Autodesk Fusion 360 part; units mm, degrees
sketch "Sketch1" plane through (0, 0, 0) normal (0, 0, 1) x (1, 0, 0) in component "Upper Layer"
  line L0 (30, -35) -> (-30, -35)
  line L1 (-30, -35) -> (-30, 35)
  line L2 (-30, 35) -> (30, 35)
  line L3 (30, 35) -> (30, -35)
  line L4 (30, -35) -> (-30, 35) construction
  line L5 (-30, -35) -> (30, 35) construction
  line L6 (28, -38) -> (-28, -38)
  line L7 (-33, -33) -> (-33, 33)
  line L8 (-28, 38) -> (28, 38)
  line L9 (33, 33) -> (33, -33)
  line L10 (33, -38) -> (-33, 38) construction
  line L11 (-33, -38) -> (33, 38) construction
  arc A0 (-28, 38) -> (-33, 33) centre (-28, 33) ccw
  arc A1 (33, 33) -> (28, 38) centre (28, 33) ccw
  arc A2 (-33, -33) -> (-28, -38) centre (-28, -33) ccw
  arc A3 (28, -38) -> (33, -33) centre (28, -33) ccw
  dimension "d1" = 60
  dimension "d2" = 70
  dimension "d3" = 66
  dimension "d4" = 76
  dimension "d51" = 5
  dimension "d52" = 5
  dimension "d53" = 5
  dimension "d54" = 5
extrude "Extrude1" add sketch "Sketch1" along normal blind 3 contours L0 L1 L2 L3 | L6 L7 L8 L9 A0 A1 A2 A3 in component "Upper Layer"
sketch "Sketch2" plane through (0, 0, 3) normal (0, 0, 1) x (-1, 0, 0) in component "Upper Layer"
  line L0 (-28, -38) -> (28, -38)
  line L1 (33, -33) -> (33, 33)
  line L2 (28, 38) -> (-28, 38)
  line L3 (-33, 33) -> (-33, -33)
  line L4 (-30, 35) -> (30, 35)
  line L5 (30, 35) -> (30, -35)
  line L6 (30, -35) -> (-30, -35)
  line L7 (-30, -35) -> (-30, 35)
  line L8 (-30, 35) -> (30, -35) construction
  line L9 (30, 35) -> (-30, -35) construction
  line L10 (0, 35) -> (0, -35) construction
  line L11 (2.5, -11) -> (-2.5, -11)
  line L12 (-2.5, -11) -> (-2.5, -20)
  line L13 (-2.5, -20) -> (2.5, -20)
  line L14 (2.5, -20) -> (2.5, -11)
  line L15 (2.5, -11) -> (-2.5, -20) construction
  line L16 (-2.5, -11) -> (2.5, -20) construction
  line L17 (0, -11) -> (0, 9) construction
  line L18 (0, 9) -> (-7.5, 9) construction
  line L19 (-7.5, 9) -> (-15.5, 9)
  line L20 (-15.5, 9) -> (-15.5, 4)
  line L21 (-15.5, 4) -> (-7.5, 4)
  line L22 (-7.5, 4) -> (-7.5, 9)
  line L23 (15.5, 4) -> (7.5, 4)
  line L24 (7.5, 4) -> (7.5, 9)
  line L25 (15.5, 9) -> (15.5, 4)
  line L26 (7.5, 9) -> (15.5, 9)
  line L27 (-5.5, -8) -> (5.5, -8)
  line L28 (5.5, -8) -> (5.5, -23)
  line L29 (5.5, -23) -> (-5.5, -23)
  line L30 (-5.5, -23) -> (-5.5, -8)
  line L31 (-5.5, -8) -> (5.5, -23) construction
  line L32 (5.5, -8) -> (-5.5, -23) construction
  line L33 (-11.5, 9) -> (-11.5, 4) construction
  line L34 (-7.5, 6.5) -> (-15.5, 6.5) construction
  line L35 (-19, 11.5) -> (-4, 11.5)
  line L36 (-4, 11.5) -> (-4, 1.5)
  line L37 (-4, 1.5) -> (-19, 1.5)
  line L38 (-19, 1.5) -> (-19, 11.5)
  line L39 (-19, 11.5) -> (-4, 1.5) construction
  line L40 (-4, 11.5) -> (-19, 1.5) construction
  line L41 (4, 1.5) -> (19, 1.5)
  line L42 (4, 11.5) -> (4, 1.5)
  line L43 (19, 11.5) -> (4, 11.5)
  line L44 (19, 1.5) -> (19, 11.5)
  arc A0 (33, 33) -> (28, 38) centre (28, 33) ccw
  arc A1 (-28, 38) -> (-33, 33) centre (-28, 33) ccw
  arc A2 (-33, -33) -> (-28, -38) centre (-28, -33) ccw
  arc A3 (28, -38) -> (33, -33) centre (28, -33) ccw
  point P0 (0, -15.5)
  point P1 (0, -15.5)
  point P2 (-11.5, 6.5)
  dimension "d7" = 5
  dimension "d8" = 9
  dimension "d9" = 20
  dimension "d10" = 7.5
  dimension "d11" = 8
  dimension "d12" = 5
  dimension "d13" = 11
  dimension "d14" = 15
  dimension "d15" = 15
  dimension "d16" = 10
extrude "Extrude2" cut sketch "Sketch2" against normal up to surface (3 mm away) contours L11 L12 L13 L14 in component "Upper Layer"
extrude "Extrude3" add sketch "Sketch2" along normal blind 3 contours L27 L28 L29 L30 in component "Upper Layer"
extrude "Extrude4" cut sketch "Sketch2" against normal up to surface (3 mm away) contours L19 L20 L21 L22 | L23 L24 L25 L26 in component "Upper Layer"
extrude "Extrude5" add sketch "Sketch2" along normal blind 3 contours L35 L36 L37 L38 | L41 L42 L43 L44 in component "Upper Layer"
sketch "Sketch2 (2)" plane through (0, 0, -8.9199) normal (0, 0, -1) x (1, 0, 0)
  line L0 (22.45, -32.5) -> (22.45, -27.6)
  line L1 (22.45, -27.6) -> (17.55, -27.6)
  line L2 (17.55, -27.6) -> (17.55, -32.5)
  line L3 (17.55, -32.5) -> (22.45, -32.5)
  line L4 (-17.55, -32.45) -> (-17.55, -27.55)
  line L5 (-17.55, -27.55) -> (-22.45, -27.55)
  line L6 (-22.45, -27.55) -> (-22.45, -32.45)
  line L7 (-22.45, -32.45) -> (-17.55, -32.45)
sketch "Sketch4" plane through (0, 0, 3) normal (0, 0, 1) x (1, 0, 0) in component "Upper Layer"
  line L0 (0, 30) -> (-18, 30) construction
  circle A0 centre (-18, 30) radius 3
  line L1 (-18, 30) -> (-15, 30)
  line L2 (-18, 30) -> (-7.5877, 30) construction
  line L3 (-18, 30) -> (18, 30) construction
  circle A1 centre (18, 30) radius 3
  dimension "d37" = 6
  dimension "d38" = 36
  dimension "d39" = 6
  dimension "d50" = 18
extrude "Extrude9" cut sketch "Sketch4" against normal up to surface (3 mm away) in component "Upper Layer"
sketch "Sketch3" plane through (0, 0, 3) normal (0, 0, 1) x (-1, 0, 0)
  line L0 (30, 35) -> (27.5, 35) construction
  line L1 (30, 35) -> (30, 32.5) construction
  circle A0 centre (27.5, 32.5) radius 2.5
  line L2 (40, 0) -> (-40, 0)
  line L3 (0, -45) -> (0, 47.452)
  circle A1 centre (27.5, -32.5) radius 2.5
  circle A2 centre (-27.5, -32.5) radius 2.5
  circle A3 centre (-27.5, 32.5) radius 2.5
  circle A4 centre (27.5, -32.5) radius 1.5
  circle A5 centre (27.5, 32.5) radius 1.5
  circle A6 centre (-27.5, -32.5) radius 1.5
  circle A7 centre (-27.5, 32.5) radius 1.5
  dimension "d42" = 2.5
  dimension "d43" = 2.5
  dimension "d44" = 3
  dimension "d45" = 3
  dimension "d46" = 3
  dimension "d47" = 3
extrude "Extrude10" cut sketch "Sketch3" against normal blind 3 contours A4 | A5 | A6 | A7 in component "Upper Layer"
component "Upper Layer" placed x (1, 0, 0) y (0, 1, 0) z (0, 0, 1) at (0, 0, 0)
equation "d10 = ( 15 / 2 ) * 1 mm"
Part model, mm, in its own coordinate system. A direction names the side the tool comes from. Round coordinates to 2 decimals unless told otherwise and drop trailing zeros. Write each loop counter-clockwise with the first axis right and the second up, starting at its lowest first coordinate (ties: lowest second). Pieces come first, ordered by that corner, then holes.
Item 1: Probe L1, parallel to X at y = -5.5, z = 5.5; L2, parallel to Y at x = -27.5, z = 0.9; L3, parallel to X at y = 19, z = 3.7. List the from-to ranges inside material, lowest first.
Results:
L1: x = -19 to -15.5, -7.5 to -4, 4 to 7.5, 15.5 to 19
L2: y = -38 to -34, -31 to 31, 34 to 38
L3: x = -5.5 to -2.5, 2.5 to 5.5
Item 2: Cut at C-C, the plane y = 30. Give the cut face in (x, z), plus the area to 3 significant figures.
Results:
outline: (-33, 0) - (-21, 0) - (-21, 3) - (-33, 3) - close; (-15, 0) - (15, 0) - (15, 3) - (-15, 3) - close; (21, 0) - (33, 0) - (33, 3) - (21, 3) - close
area: 162 mm2
Item 3: Two-plate mould, pull along X, no slides. Class faces 1 (the flat face through (0, 38, 1)), 2 (the cylindrical face through (-26.3, 33.4, 1.5)), 3 (the cylindrical face through (-26.3, -31.6, 1.5)), 4 (the flat face through (5.5, 16, 4)): +X half, -X half, draft (parallel to the pull), parting line (faces both ways), or undercut.
Results:
face 1: draft
face 2: undercut
face 3: undercut
face 4: +X half
Item 4: Cut at A-A, the plane x = 18. Give the cut face in (y, z), plus the area to 3 significant figures.
Results:
outline: (-38, 0) - (27, 0) - (27, 3) - (-1.5, 3) - (-1.5, 6) - (-11.5, 6) - (-11.5, 3) - (-38, 3) - close; (33, 0) - (38, 0) - (38, 3) - (33, 3) - close
area: 240 mm2
Item 5: Drop flat-ended pins along their axis: pin 1 Ø1.5 at (x, z) = (-14.5, 5) entering from -Y; pin 2 Ø5 at (x, y) = (-27.5, -32.5) entering from -Z; pin 3 Ø8 at (x, y) = (-3.5, -18.5) entering from +Z; pin 4 Ø3.5 at (x, z) = (1, 5) entering from -Y. Give the stop position or say it passes through.
Results:
pin 1: stops at y = -11.5
pin 2: stops at z = 0
pin 3: stops at z = 3
pin 4: stops at y = 8
Item 6: Cut at B-B, the plane z = 1.55. Count the separate pieces of the cut face and the enclosed holes in it, plus the area to 3 significant figures.
Results:
separate pieces: 1
enclosed holes: 9
area: 4,780 mm2
Item 7: Which spindle directions (+Z, -Z, +X, -X, +Y, -Y) get a long thin tool onto all of the face, cutting with end or side? Do faces 5 (the flat face through (0, 23, 4)), 6 (the flat face through (-19, -6, 4)), 7 (the flat face through (-12, -11.5, 4)), 8 (the flat face through (-33, 0, 1)), 9 (the flat face through (0, 20, 3)). Say none if no direction does.
Results:
face 5: +Z, +X, -X, +Y
face 6: +Z, -X, +Y, -Y
face 7: +Z, +X, -X, -Y
face 8: +Z, -Z, -X, +Y, -Y
face 9: +Z, -Z
Item 8: Cut at D-D, the plane x = -0.5. Give the cut face in (y, z), plus the area to 3 significant figures.
Results:
outline: (-38, 0) - (11, 0) - (11, 6) - (8, 6) - (8, 3) - (-38, 3) - close; (20, 0) - (38, 0) - (38, 3) - (23, 3) - (23, 6) - (20, 6) - close
area: 219 mm2
